Geometry: see drawing. Coordinates: mm, zero at the bounding-box minimum. A direction names the side the tool comes from. Coordinates: 2 decimals unless noted, no trailing zeros. Loops run counter-clockwise (first coordinate to the right, second up) from the corner with the lowest first, then second, coordinate; pieces in that order, holes last. Notation, with made-up numbers: (-29.5, 30) -> (23.5, 30) arc R20 cw to (23.5, 62) -> close; hole circle Ø1 at (-8.5, -8). An arc over 180 degrees is marked (long way). One line per question, with ' | ' between items. Start each with the question number.
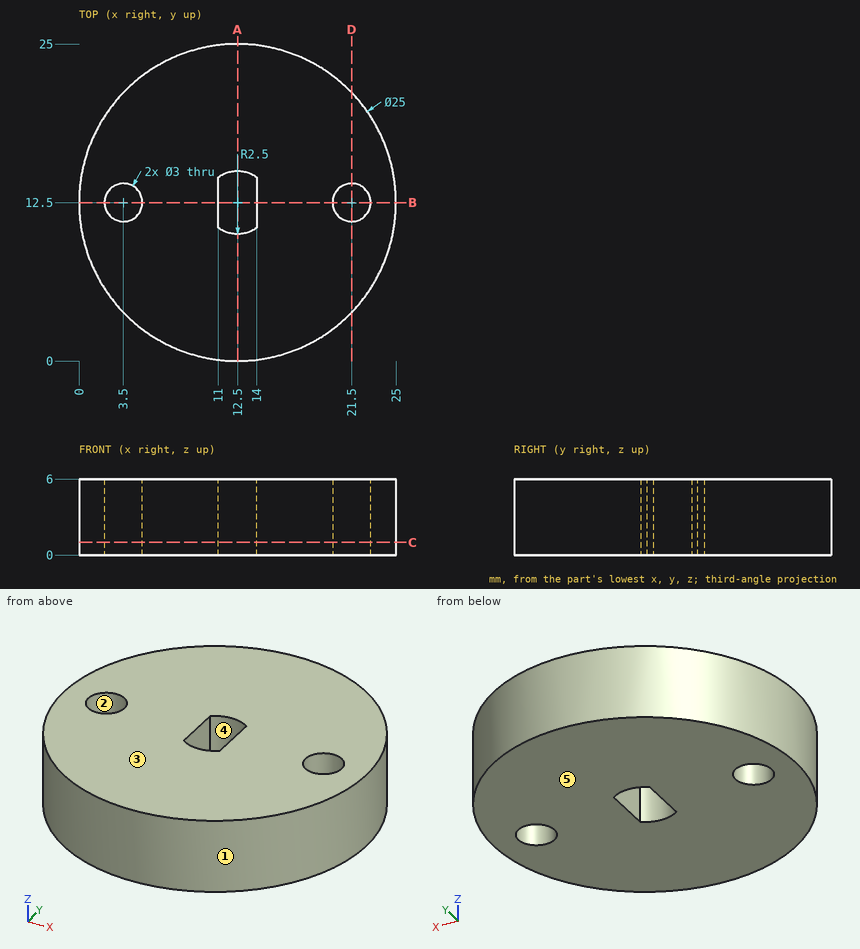
(1) Cut plane A-A, the plane x = 12.5. Return the cut outline in (y, z), and give its area (3 significant figures).
(2) Contact query for flat-ended pins moving along their axis: pin 1 Ø1 at (x, z) = (14.5, 1) entering from +Y; pin 2 Ø1.5 at (x, z) = (21.5, 5) entering from -Y; pin 3 Ø1.5 at (x, z) = (4.5, 2.5) entering from +Y. Output: stop coordinate, or through.
(3) Ray query, L1, parallel to X at y = 12.25, z = 0.5; L2, parallel to X at y = 11.25, z = 5.4; L3, parallel to Y at x = 3, z = 4.35. Return the intervals inside material, ascending.
(4) Cut plane B-B, the plane y = 12.5. Return the cut outline in (x, z), and give its area (3 significant figures).
(5) Cut plane C-C, the plane z = 1. Return the cut outline in (x, y).
(6) Access query for the marked faces 4 and 5. Directions: +Z, -Z, +X, -X, +Y, -Y. A direction counts if a zero-diameter tool reaches every point of the face in a straight line with its end or side. Return the directions, or none.
(7) Draft query along Y for the marked faces 1, 2 and 3. Return one class per face: pulls with the +Y half, pulls with the -Y half, needs draft (parallel to the pull), parting line crosses it, or undercut.
(8) Cut plane D-D, the plane x = 21.5. Return the cut outline in (y, z).
Here are the results:
1) outline: (0, 0) -> (10, 0) -> (10, 6) -> (0, 6) -> close; (15, 0) -> (25, 0) -> (25, 6) -> (15, 6) -> close | area: 120 mm2
2) pin 1: stops at y = 24.91 | pin 2: stops at y = 3.11 | pin 3: stops at y = 22.68
3) L1: x = 0 to 2.02, 4.98 to 11, 14 to 20.02, 22.98 to 25 | L2: x = 0.06 to 2.67, 4.33 to 11, 14 to 20.67, 22.33 to 24.94 | L3: y = 4.38 to 11.09, 13.91 to 20.62
4) outline: (0, 0) -> (2, 0) -> (2, 6) -> (0, 6) -> close; (5, 0) -> (11, 0) -> (11, 6) -> (5, 6) -> close; (14, 0) -> (20, 0) -> (20, 6) -> (14, 6) -> close; (23, 0) -> (25, 0) -> (25, 6) -> (23, 6) -> close | area: 96.0 mm2
5) outline: circle Ø25 at (12.5, 12.5); hole circle Ø3 at (3.5, 12.5); hole (11, 10.5) arc R2.5 ccw to (14, 10.5) -> (14, 14.5) arc R2.5 ccw to (11, 14.5) -> close; hole circle Ø3 at (21.5, 12.5)
6) face 4: +Z, -Z | face 5: -Z, +X, -X, +Y, -Y
7) face 1: parting line crosses it | face 2: undercut | face 3: needs draft
8) outline: (3.83, 0) -> (11, 0) -> (11, 6) -> (3.83, 6) -> close; (14, 0) -> (21.17, 0) -> (21.17, 6) -> (14, 6) -> close
